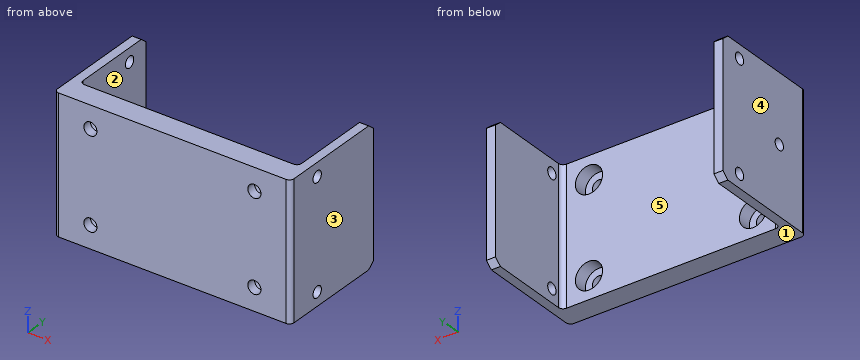
```python
from build123d import *
from OCP.BRepFilletAPI import BRepFilletAPI_MakeChamfer

# Parameters (mm, degrees)
SKETCH1_W           = 52.2
SKETCH1_H           = 30
BOSS_EXTRUDE1_DEPTH = 3
SKETCH2_W           = 2
SKETCH2_H           = 30
BOSS_EXTRUDE2_DEPTH = 20
SKETCH3_W           = 2
SKETCH3_H           = 30
BOSS_EXTRUDE3_DEPTH = 20
SKETCH4_R           = 1.252611376
SKETCH4_R_2         = 1.250208487
CUT_EXTRUDE2_DEPTH  = 5
SKETCH5_R           = 1.25
SKETCH5_R_2         = 1.249999994
CUT_EXTRUDE4_DEPTH  = 5
SKETCH6_R           = 3
CUT_EXTRUDE5_DEPTH  = 3
SKETCH7_W           = 52.2
SKETCH7_H           = 30
BOSS_EXTRUDE4_DEPTH = 2
SKETCH8_R           = 1.45
CUT_EXTRUDE6_DEPTH  = 2
FILLET1_R           = 1
CHAMFER2_SIZE       = 1.5
CHAMFER2_SIZE2      = 1.258649447


with BuildPart() as part:
    # Sketch1 → Boss-Extrude1 (new body)
    with BuildSketch(Plane(origin=(0, 0, 0), x_dir=(1, 0, 0), z_dir=(0, 1, 0))):
        Rectangle(SKETCH1_W, SKETCH1_H)
    extrude(amount=BOSS_EXTRUDE1_DEPTH)

    # Sketch2 → Boss-Extrude2 (add)
    with BuildSketch(Plane(origin=(0, 3, 0), x_dir=(1, 0, 0), z_dir=(0, 1, 0))):
        with Locations((-25.1, 0)):
            Rectangle(SKETCH2_W, SKETCH2_H)
    extrude(amount=BOSS_EXTRUDE2_DEPTH)

    # Sketch3 → Boss-Extrude3 (add)
    with BuildSketch(Plane(origin=(0, 3, 0), x_dir=(1, 0, 0), z_dir=(0, 1, 0))):
        with Locations((25.1, 0)):
            Rectangle(SKETCH3_W, SKETCH3_H)
    extrude(amount=BOSS_EXTRUDE3_DEPTH)

    # Sketch4 → Cut-Extrude2 (cut)
    with BuildSketch(Plane(origin=(26.1, 0, 0), x_dir=(0, 0, -1), z_dir=(1, 0, 0))):
        with Locations((12, 6)):
            Circle(SKETCH4_R)
        with Locations((-12, 6)):
            Circle(SKETCH4_R_2)
    extrude(amount=-CUT_EXTRUDE2_DEPTH, mode=Mode.SUBTRACT)

    # Sketch5 → Cut-Extrude4 (cut)
    with BuildSketch(Plane(origin=(-24.1, 0, 0), x_dir=(0, 0, -1), z_dir=(1, 0, 0))):
        with Locations((-12.00000002, 18)):
            Circle(SKETCH5_R)
        with Locations((12.00000002, 18)):
            Circle(SKETCH5_R)
        with Locations((0, 6)):
            Circle(SKETCH5_R_2)
    extrude(amount=-CUT_EXTRUDE4_DEPTH, mode=Mode.SUBTRACT)

    # Sketch6 → Cut-Extrude5 (cut)
    with BuildSketch(Plane(origin=(0, 3, 0), x_dir=(1, 0, 0), z_dir=(0, 1, 0))):
        with Locations(Location((-18.1, 10, 0), (0, 0, 270))):
            Circle(SKETCH6_R)
        with Locations(Location((-18.1, -10, 0), (0, 0, 270))):
            Circle(SKETCH6_R)
        with Locations(Location((18.1, 10, 0), (0, 0, 270))):
            Circle(SKETCH6_R)
        with Locations(Location((18.1, -10, 0), (0, 0, 270))):
            Circle(SKETCH6_R)
    extrude(amount=-CUT_EXTRUDE5_DEPTH, mode=Mode.SUBTRACT)

    # Sketch7 → Boss-Extrude4 (add)
    with BuildSketch(Plane.XZ):
        Rectangle(SKETCH7_W, SKETCH7_H)
    extrude(amount=BOSS_EXTRUDE4_DEPTH)

    # Sketch8 → Cut-Extrude6 (cut)
    with BuildSketch(Plane(origin=(0, 0, 0), x_dir=(1, 0, 0), z_dir=(0, 1, 0))):
        with Locations(Location((-18.1, 10, 0), (0, 0, 270))):
            Circle(SKETCH8_R)
        with Locations(Location((18.1, 10, 0), (0, 0, 270))):
            Circle(SKETCH8_R)
        with Locations(Location((18.1, -10, 0), (0, 0, 270))):
            Circle(SKETCH8_R)
        with Locations(Location((-18.1, -10, 0), (0, 0, 270))):
            Circle(SKETCH8_R)
    extrude(amount=-CUT_EXTRUDE6_DEPTH, mode=Mode.SUBTRACT)

    # Fillet1
    fillet1_edges = [part.edges().sort_by_distance(p)[0] for p in [
        (-24.1, 3, 0),
        (24.1, 3, 0),
        (-26.1, -2, 0),
        (26.1, -2, 0),
    ]]
    fillet(fillet1_edges, radius=FILLET1_R)

    # Chamfer2: one chamfer whose edges measure the first distance from different faces: ONE call of the kernel's chamfer builder (chamfer() names one face for all edges)
    chamfer2_edges_1 = [part.edges().sort_by_distance(p)[0] for p in [
        (-25.1, 23, 15),
        (25.1, 23, 15),
    ]]
    chamfer2_side_1 = [part.faces().sort_by_distance(p)[0] for p in [
        (-25.521221977, 11, 15),
    ]]
    chamfer2_edges_2 = [part.edges().sort_by_distance(p)[0] for p in [
        (-25.1, 23, -15),
        (25.1, 23, -15),
    ]]
    chamfer2_side_2 = [part.faces().sort_by_distance(p)[0] for p in [
        (24.678778023, 13.5, -15),
    ]]
    chamfer2 = BRepFilletAPI_MakeChamfer(part.part.solid().wrapped)
    for e in chamfer2_edges_1:
        chamfer2.Add(CHAMFER2_SIZE, CHAMFER2_SIZE2, e.wrapped, chamfer2_side_1[0].wrapped)  # the first distance lies on this face
    for e in chamfer2_edges_2:
        chamfer2.Add(CHAMFER2_SIZE, CHAMFER2_SIZE2, e.wrapped, chamfer2_side_2[0].wrapped)  # the first distance lies on this face
    add(Compound.cast(chamfer2.Shape()), mode=Mode.REPLACE)


solid = part.part
```
Geometry check sheet. Reference: the model listing, model coordinates, mm. Face numbers are marked on the shaded views. A direction names the side the tool comes from. Round coordinates to 2 decimals unless told otherwise and drop trailing zeros. Loops run counter-clockwise (first coordinate to the right, second up) from the corner with the lowest first, then second, coordinate; pieces in that order, holes last. Notation, with made-up numbers: (72, -8) -> (112, -8) arc R35 ccw to (112, 31) -> close; hole circle Ø2 at (45, -26.5). An arc over 180 degrees is marked (long way). Use a Markdown table: item, result.
(1) Go/stop test with flat-tipped pins: P1, Ø2.5, axis at x = 18.1, z = -10, coming from the -Y side; P2, Ø15, axis at x = -10.5, z = -1, coming from the +Y side. Record where each tip stops, or that it passes through.
Calculated:
| item | result |
|---|---|
| P1 | through |
| P2 | y = 3 |
(2) Sectioned sample at B-B (z = 0). Enter the section's corners in (x, y), then the cut area to 3 significant figures.
Calculated:
| item | result |
|---|---|
| outline | (-26.1, -1) arc R1 ccw to (-25.1, -2) -> (25.1, -2) arc R1 ccw to (26.1, -1) -> (26.1, 23) -> (24.1, 23) -> (24.1, 4) arc R1 cw to (23.1, 3) -> (-23.1, 3) arc R1 cw to (-24.1, 4) -> (-24.1, 4.75) -> (-26.1, 4.75) -> close; (-26.1, 7.25) -> (-24.1, 7.25) -> (-24.1, 23) -> (-26.1, 23) -> close |
| area | 336 mm² |
(3) Scan lines: probe 1 along X at (y, z) = (-0.8, -10); probe 2 along X at (y, z) = (2.1, -10); probe 3 along X at (y, z) = (21.25, 13). Record each from-to range of solid material in increasing order.
Calculated:
| item | result |
|---|---|
| probe 1 | -26.1 to -19.55, -16.65 to 16.65, 19.55 to 26.1 |
| probe 2 | -26.1 to -21.1, -15.1 to 15.1, 21.1 to 26.1 |
| probe 3 | -26.1 to -24.1, 24.1 to 26.1 |
(4) Mould release check, pull along X, two halves, no side actions. Record for the marked faces 1, 2 and 3: released by +X, released by -X, zero draft, split by the parting line, or undercut.
Calculated:
| item | result |
|---|---|
| face 1 | zero draft |
| face 2 | undercut |
| face 3 | released by +X |
(5) Sectioned sample at D-D (y = 6). Enter the section's corners in (x, z), then the cut area to 3 significant figures.
Calculated:
| item | result |
|---|---|
| outline | (-26.1, -15) -> (-24.1, -15) -> (-24.1, -1.25) -> (-26.1, -1.25) -> close; (-26.1, 1.25) -> (-24.1, 1.25) -> (-24.1, 15) -> (-26.1, 15) -> close; (24.1, -15) -> (26.1, -15) -> (26.1, -13.25) -> (24.1, -13.25) -> close; (24.1, -10.75) -> (26.1, -10.75) -> (26.1, 10.75) -> (24.1, 10.75) -> close; (24.1, 13.25) -> (26.1, 13.25) -> (26.1, 15) -> (24.1, 15) -> close |
| area | 105 mm² |
(6) Sectioned sample at C-C (x = -18.1). Enter the section's corners in (y, z), then the cut area to 3 significant figures.
Calculated:
| item | result |
|---|---|
| outline | (-2, -15) -> (3, -15) -> (3, -13) -> (0, -13) -> (0, -11.45) -> (-2, -11.45) -> close; (-2, -8.55) -> (0, -8.55) -> (0, -7) -> (3, -7) -> (3, 7) -> (0, 7) -> (0, 8.55) -> (-2, 8.55) -> close; (-2, 11.45) -> (0, 11.45) -> (0, 13) -> (3, 13) -> (3, 15) -> (-2, 15) -> close |
| area | 102 mm² |
(7) Set-up check for the marked faces 4 and 5: record each of +Z, -Z, +X, -X, +Y, -Y from which the full face is reachable in a straight line by a thin tool's end or side.
Calculated:
| item | result |
|---|---|
| face 4 | +Z, -Z, -X, +Y, -Y |
| face 5 | +Z, -Z, +Y |
(8) Sectioned sample at A-A (y = 18). Enter the section's corners in (x, z).
Calculated:
| item | result |
|---|---|
| outline | (-26.1, -15) -> (-24.1, -15) -> (-24.1, -13.25) -> (-26.1, -13.25) -> close; (-26.1, -10.75) -> (-24.1, -10.75) -> (-24.1, 10.75) -> (-26.1, 10.75) -> close; (-26.1, 13.25) -> (-24.1, 13.25) -> (-24.1, 15) -> (-26.1, 15) -> close; (24.1, -15) -> (26.1, -15) -> (26.1, 15) -> (24.1, 15) -> close |
